```python
from build123d import *

# Parameters (mm, degrees)
SKETCH_1_W          = 140
SKETCH_1_H          = 124
EXTRUDE_1_DEPTH     = 0.5
CUT_EXTRUDE_1_DEPTH = 1.5
SKETCH_3_W          = 12
SKETCH_3_H          = 40
EXTRUDE_2_DEPTH     = 1
SKETCH_5_R          = 1.525
CUT_EXTRUDE_3_DEPTH = 10
FILLET_1_R          = 1.5
SKETCH_8_W          = 26.5
SKETCH_8_H          = 5
CUT_EXTRUDE_5_DEPTH = 10
CUT_EXTRUDE_6_DEPTH = 10
CUT_EXTRUDE_7_DEPTH = 10
FILLET_2_R          = 2
FILLET_3_R          = 1
FILLET_4_R          = 1
CUT_EXTRUDE_8_DEPTH = 5


with BuildPart() as part:
    # 草图1 → 凸台-拉伸1 (new, symmetric)
    with BuildSketch(Plane.XY):
        Rectangle(SKETCH_1_W, SKETCH_1_H)
    extrude(amount=EXTRUDE_1_DEPTH, both=True)

    # 草图2 → 切除-拉伸1 (cut, symmetric)
    with BuildSketch(Plane.XY.offset(0.5)):
        Polygon((-0.3, -62), (-0.3, -24), (56.860254038, -24), (33.816623489, 62), (70, 62), (70, -62), align=None)
    extrude(amount=CUT_EXTRUDE_1_DEPTH, both=True, mode=Mode.SUBTRACT)

    # 草图3 → 凸台-拉伸2 (add)
    with BuildSketch(Plane.XY.offset(0.5)):
        with Locations((-70, 22)):
            Rectangle(SKETCH_3_W, SKETCH_3_H)
    extrude(amount=-EXTRUDE_2_DEPTH)

    # 草图5 → 切除-拉伸3 (cut)
    with BuildSketch(Plane(origin=(0, 0, -0.5), x_dir=(-1, 0, 0), z_dir=(0, 0, -1))):
        with Locations((34.915427319, 58)):
            Circle(SKETCH_5_R)
        with Locations((54.915427319, 58)):
            Circle(SKETCH_5_R)
        with Locations((73, 27)):
            Circle(SKETCH_5_R)
        with Locations((73, 7)):
            Circle(SKETCH_5_R)
    extrude(amount=-CUT_EXTRUDE_3_DEPTH, mode=Mode.SUBTRACT)

    # 圆角1
    fillet_1_edges = [part.edges().sort_by_distance(p)[0] for p in [
        (-0.3, -62, 0),
        (-0.3, -24, 0),
        (56.860254038, -24, 0),
        (33.816623489, 62, 0),
        (-76, 42, 0),
        (-70, 42, 0),
        (-76, 2, 0),
        (-70, 2, 0),
        (-70, -62, 0),
        (-70, 62, 0),
    ]]
    fillet(fillet_1_edges, radius=FILLET_1_R)

    # 草图8 → 切除-拉伸5 (cut)
    with BuildSketch(Plane(origin=(0, 0, -0.5), x_dir=(-1, 0, 0), z_dir=(0, 0, -1))):
        with Locations((12.05, -26.5)):
            Rectangle(SKETCH_8_W, SKETCH_8_H)
    extrude(amount=-CUT_EXTRUDE_5_DEPTH, mode=Mode.SUBTRACT)

    # 草图9 → 切除-拉伸6 (cut)
    with BuildSketch(Plane(origin=(0, 0, -0.5), x_dir=(-1, 0, 0), z_dir=(0, 0, -1))):
        with BuildLine():
            Line((23.15, -41.85), (31.15, -41.85))
            ThreePointArc((31.15, -41.85), (32.3, -43), (31.15, -44.15))
            Line((31.15, -44.15), (23.15, -44.15))
            ThreePointArc((23.15, -44.15), (22, -43), (23.15, -41.85))
        make_face()
        with BuildLine():
            Line((7.15, -41.85), (15.15, -41.85))
            ThreePointArc((15.15, -41.85), (16.3, -43), (15.15, -44.15))
            Line((15.15, -44.15), (7.15, -44.15))
            ThreePointArc((7.15, -44.15), (6, -43), (7.15, -41.85))
        make_face()
        with BuildLine():
            Line((47.15, -41.85), (39.15, -41.85))
            ThreePointArc((39.15, -41.85), (38, -43), (39.15, -44.15))
            Line((39.15, -44.15), (47.15, -44.15))
            ThreePointArc((47.15, -44.15), (48.3, -43), (47.15, -41.85))
        make_face()
        with BuildLine():
            Line((63.15, -41.85), (55.15, -41.85))
            ThreePointArc((55.15, -41.85), (54, -43), (55.15, -44.15))
            Line((55.15, -44.15), (63.15, -44.15))
            ThreePointArc((63.15, -44.15), (64.3, -43), (63.15, -41.85))
        make_face()
        with BuildLine():
            Line((23.15, -56.15), (31.15, -56.15))
            ThreePointArc((31.15, -56.15), (32.3, -55), (31.15, -53.85))
            Line((31.15, -53.85), (23.15, -53.85))
            ThreePointArc((23.15, -53.85), (22, -55), (23.15, -56.15))
        make_face()
        with BuildLine():
            Line((7.15, -56.15), (15.15, -56.15))
            ThreePointArc((15.15, -56.15), (16.3, -55), (15.15, -53.85))
            Line((15.15, -53.85), (7.15, -53.85))
            ThreePointArc((7.15, -53.85), (6, -55), (7.15, -56.15))
        make_face()
        with BuildLine():
            Line((47.15, -56.15), (39.15, -56.15))
            ThreePointArc((39.15, -56.15), (38, -55), (39.15, -53.85))
            Line((39.15, -53.85), (47.15, -53.85))
            ThreePointArc((47.15, -53.85), (48.3, -55), (47.15, -56.15))
        make_face()
        with BuildLine():
            Line((63.15, -56.15), (55.15, -56.15))
            ThreePointArc((55.15, -56.15), (54, -55), (55.15, -53.85))
            Line((55.15, -53.85), (63.15, -53.85))
            ThreePointArc((63.15, -53.85), (64.3, -55), (63.15, -56.15))
        make_face()
    extrude(amount=-CUT_EXTRUDE_6_DEPTH, mode=Mode.SUBTRACT)

    # 草图10 → 切除-拉伸7 (cut)
    with BuildSketch(Plane.XY.offset(0.5)):
        Polygon((1.02106128, 59.531168527), (1.02106128, 62), (-29.703905389, 62), (-9.798233064, 47), align=None)
    extrude(amount=-CUT_EXTRUDE_7_DEPTH, mode=Mode.SUBTRACT)

    # 圆角2
    fillet_2_edges = [part.edges().sort_by_distance(p)[0] for p in [
        (1.02106128, 59.531168527, 0),
        (-9.798233064, 47, 0),
    ]]
    fillet(fillet_2_edges, radius=FILLET_2_R)

    # 圆角3
    fillet_3_edges = [part.edges().sort_by_distance(p)[0] for p in [
        (-29.703905389, 62, 0),
        (1.02106128, 62, 0),
    ]]
    fillet(fillet_3_edges, radius=FILLET_3_R)

    # 圆角4
    fillet_4_edges = [part.edges().sort_by_distance(p)[0] for p in [
        (-25.3, -24, 0),
        (-25.3, -29, 0),
    ]]
    fillet(fillet_4_edges, radius=FILLET_4_R)

    # 草图11 → 切除-拉伸8 (cut, symmetric)
    with BuildSketch(Plane(origin=(0, 0, -0.5), x_dir=(-1, 0, 0), z_dir=(0, 0, -1))):
        with BuildLine():
            Line((-29.343347144, 59.5), (-23.343347144, 59.5))
            ThreePointArc((-23.343347144, 59.5), (-22.343347144, 58.5), (-23.343347144, 57.5))
            Line((-23.343347144, 57.5), (-29.343347144, 57.5))
            ThreePointArc((-29.343347144, 57.5), (-30.343347144, 58.5), (-29.343347144, 59.5))
        make_face()
        with BuildLine():
            Line((-5.343347144, 59.5), (-11.343347144, 59.5))
            ThreePointArc((-11.343347144, 59.5), (-12.343347144, 58.5), (-11.343347144, 57.5))
            Line((-11.343347144, 57.5), (-5.343347144, 57.5))
            ThreePointArc((-5.343347144, 57.5), (-4.343347144, 58.5), (-5.343347144, 59.5))
        make_face()
    extrude(amount=CUT_EXTRUDE_8_DEPTH, both=True, mode=Mode.SUBTRACT)


solid = part.part
```
Can you work these out from the model? Positions are in its coordinate system, mm. A direction names the side the tool comes from. Coordinates: 2 decimals unless noted, no trailing zeros. Order: outer loops, then holes, each group sorted by start corner. A loop starts at its lowest first (then second) coordinate and runs counter-clockwise, first axis right, second up. Notation, with made-up numbers: (48.5, -34) - (70.5, -34) arc R25 cw to (70.5, 0) - close; hole circle Ø1 at (40, -38.5). An arc over 180 degrees is marked (long way). Answer in a Markdown table with one row per item.
1. Suppose I cut it at A-A (x = -73). Please give me the cut outline in (y, z) (3 decimals), and give its area (3 significant figures).
Reply:
| item | result |
|---|---|
| outline | (2, -0.5) - (5.475, -0.5) - (5.475, 0.5) - (2, 0.5) - close; (8.525, -0.5) - (25.475, -0.5) - (25.475, 0.5) - (8.525, 0.5) - close; (28.525, -0.5) - (42, -0.5) - (42, 0.5) - (28.525, 0.5) - close |
| area | 33.9 mm^2 |
2. For faces 4 (the cylindrical face through (-35.735, 59.286, -0.007)), 5 (the flat face through (-20.492, 55.058, 0.007)), which set-ups out of +Z, -Z, +X, -X, +Y, -Y let a thin tool reach every point of the face, with its end or its side?
Reply:
| item | result |
|---|---|
| face 4 | +Z, -Z |
| face 5 | +Z, -Z, +Y |
3. For pin 1 (0.5 mm diameter, centred on x = -27.5, z = 0, fed in from +Y); pin 2 (3.5 mm diameter, centred on x = -73, y = 27, fed in from -Z), each with a flat end and sliding along its axis, tell me the tip position at first contact or that it passes through.
Reply:
| item | result |
|---|---|
| pin 1 | stops at y = 60.53 |
| pin 2 | stops at z = -0.5 |
4. If we mould it in two halves opening along X, with no side actions, what happens to faces 1 (the flat face through (45.39, 18.81, 0.01)), 2 (the flat face through (-4.1, 53.6, 0)), 3 (the flat face through (-25, 15, -0.5))? For each: pulls with the +X half, pulls with the -X half, needs draft (parallel to the pull), parting line crosses it, or undercut.
Reply:
| item | result |
|---|---|
| face 1 | pulls with the +X half |
| face 2 | undercut |
| face 3 | needs draft |
5. Suppose I cut it at D-D (y = 27). Please give me the cut outline in (x, z) (3 decimals), and give its area (3 significant figures).
Reply:
| item | result |
|---|---|
| outline | (-76, -0.5) - (-74.525, -0.5) - (-74.525, 0.5) - (-76, 0.5) - close; (-71.475, -0.5) - (43.195, -0.5) - (43.195, 0.5) - (-71.475, 0.5) - close |
| area | 116 mm^2 |
6. Suppose I cut it at C-C (z = 0.1). Give the number of separate pieces and of enclosed holes in the cut face, and give its area (3 significant figures).
Reply:
| item | result |
|---|---|
| separate pieces | 1 |
| enclosed holes | 14 |
| area | 12,200 mm^2 |
7. Suppose I cut it at B-B (y = 7). Please give me the cut outline in (x, z) (3 decimals).
Reply:
| item | result |
|---|---|
| outline | (-76, -0.5) - (-74.525, -0.5) - (-74.525, 0.5) - (-76, 0.5) - close; (-71.475, -0.5) - (48.554, -0.5) - (48.554, 0.5) - (-71.475, 0.5) - close |
8. If I drill on line 1 along Y through (x, z) = (-73, -0.15) (3 decimals); line 2 along Y through (x, z) = (-62, -0.05); line 3 along X through (y, z) = (-35, 0.1), over which ranges is the centre line in solid material (lowest first)?
Reply:
| item | result |
|---|---|
| line 1 | y = 2 to 5.475, 8.525 to 25.475, 28.525 to 42 |
| line 2 | y = -62 to -56.15, -53.85 to -44.15, -41.85 to 62 |
| line 3 | x = -70 to -0.3 |
